The figure shows three views and two pictorial views of one solid part (mm, origin at its lowest corner). Answer the questions. Coordinates: 2 decimals unless noted, no trailing zeros. Order: outer loops, then holes, each group sorted by start corner. A loop starts at its lowest first (then second) coordinate and runs counter-clockwise, first axis right, second up. Notation, with made-up numbers: (48.5, 50) -> (57.5, 50) arc R23 cw to (57.5, 87) -> close; hole circle Ø8 at (-31, -31.75). An arc over 180 degrees is marked (long way). Return JSON: item names as keys, results as strings.
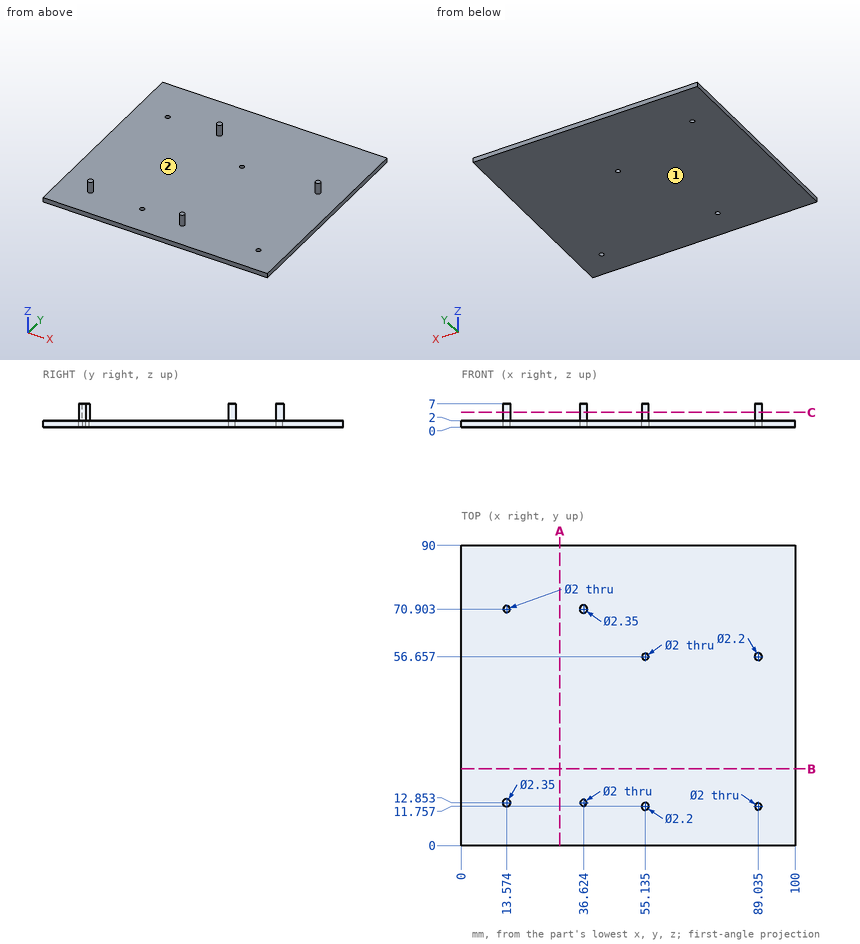
Item 1: The part is cut by section B-B on y = 23. Determine the outline of the cut face in (x, z), plus the area to 3 significant figures.
Answer list:
{"outline": "(0, 0) -> (100, 0) -> (100, 2) -> (0, 2) -> close", "area": "200 mm2"}
Item 2: The part is cut by section A-A on x = 29.5. Determine the outline of the cut face in (y, z), plus the area to 3 significant figures.
Answer list:
{"outline": "(0, 0) -> (90, 0) -> (90, 2) -> (0, 2) -> close", "area": "180 mm2"}
Item 3: Determine the mould class of the marked faces 1 and 2 for opening direction Z: pulls with the +Z half, pulls with the -Z half, needs draft (parallel to the pull), parting line crosses it, or undercut.
Answer list:
{"face 1": "pulls with the -Z half", "face 2": "pulls with the +Z half"}
Item 4: Flat-ended cylindrical pins translate along their axes: pin 1 (12 mm diameter, centred on x = 62.5, y = 67, fed in from +Z); pin 2 (1.5 mm diameter, centred on x = 48, z = 3.5, fed in from +Y). Find the tip coordinate at first contact, or state that the pin passes through.
Answer list:
{"pin 1": "z = 2", "pin 2": "through"}
Item 5: Find the intervals of material crossed by probe 1 along Z at (x, y) = (68, 48.5); probe 2 along X at (y, z) = (13, 5.75); probe 3 along Y at (x, z) = (37.5, 0.75) (1 decimal), in increasing order.
Answer list:
{"probe 1": "0 to 2", "probe 2": "12.41 to 14.74", "probe 3": "0 to 12.4, 13.3 to 90"}
Item 6: The part is cut by section C-C on z = 4.5. Count the separate pieces of the cut face and the enclosed holes in it, plus the area to 3 significant figures.
Answer list:
{"separate pieces": "4", "enclosed holes": "0", "area": "16.3 mm2"}
